Verification items for the finished model (mm, model axes). Face numbers are marked on the shaded views. A direction names the side the tool comes from. Give positions to 0.01 mm unless a question says otherwise; leave off trailing zeros. Loops run counter-clockwise (first coordinate to the right, second up) from the corner with the lowest first, then second, coordinate; pieces in that order, holes last. Notation, with made-up numbers: M 33,-6.75 L 72,-6.75 A15 ccw 72,10.25 Z; hole C 29.25,25.25 d1. An arc over 180 degrees is marked long. Answer in a Markdown table with one row per item.
```python
from build123d import *

# Parameters (mm, degrees)
SKETCH_1_W          = 30
SKETCH_1_H          = 25
SKETCH_1_W_2        = 28
SKETCH_1_H_2        = 23
EXTRUDE_1_DEPTH     = 27.5
SKETCH_2_R          = 1.5
CUT_EXTRUDE_1_DEPTH = 70
SKETCH_3_R          = 1.5
CUT_EXTRUDE_2_DEPTH = 20
SKETCH_4_R          = 1.5
CUT_EXTRUDE_3_DEPTH = 20


with BuildPart() as part:
    # 草图1 → 凸台-拉伸1 (new, symmetric)
    with BuildSketch(Plane.XY):
        Rectangle(SKETCH_1_W, SKETCH_1_H)
        Rectangle(SKETCH_1_W_2, SKETCH_1_H_2, mode=Mode.SUBTRACT)
    extrude(amount=EXTRUDE_1_DEPTH, both=True)

    # 草图2 → 切除-拉伸1 (cut)
    with BuildSketch(Plane(origin=(0, 12.5, 0), x_dir=(1, 0, 0), z_dir=(0, 1, 0))):
        with Locations(Location((0, 20, 0), (0, 0, 270))):
            Circle(SKETCH_2_R)
        with Locations(Location((0, -20, 0), (0, 0, 270))):
            Circle(SKETCH_2_R)
    extrude(amount=-CUT_EXTRUDE_1_DEPTH, mode=Mode.SUBTRACT)

    # 草图3 → 切除-拉伸2 (cut)
    with BuildSketch(Plane(origin=(-14, 0, 0), x_dir=(0, 0, -1), z_dir=(1, 0, 0))):
        Circle(SKETCH_3_R)
        with Locations((-23.5, 0)):
            Circle(SKETCH_3_R)
        with Locations((23.5, 0)):
            Circle(SKETCH_3_R)
    extrude(amount=-CUT_EXTRUDE_2_DEPTH, mode=Mode.SUBTRACT)

    # 草图4 → 切除-拉伸3 (cut)
    with BuildSketch(Plane(origin=(15, 0, 0), x_dir=(0, 0, -1), z_dir=(1, 0, 0))):
        with Locations((15, 0)):
            Circle(SKETCH_4_R)
        with Locations((-15, 0)):
            Circle(SKETCH_4_R)
    extrude(amount=-CUT_EXTRUDE_3_DEPTH, mode=Mode.SUBTRACT)


solid = part.part
```
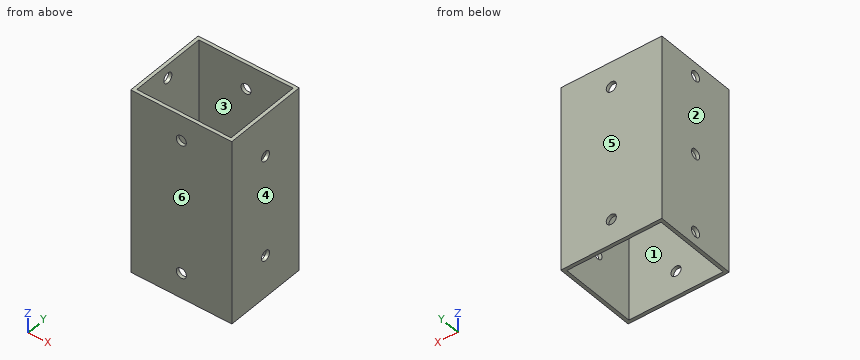
Item 1: Sectioned sample at B-B (z = -10). Record the cut outline in (x, y), and give its area (3 significant figures).
Reported:
| item | result |
|---|---|
| outline | M -15,-12.5 L 15,-12.5 L 15,12.5 L -15,12.5 Z; hole M -14,-11.5 L 14,-11.5 L 14,11.5 L -14,11.5 Z |
| area | 106 mm^2 |
Item 2: Sectioned sample at C-C (x = 5.5). Record the cut outline in (y, z), and give its area (3 significant figures).
Reported:
| item | result |
|---|---|
| outline | M -12.5,-27.5 L -11.5,-27.5 L -11.5,27.5 L -12.5,27.5 Z; M 11.5,-27.5 L 12.5,-27.5 L 12.5,27.5 L 11.5,27.5 Z |
| area | 110 mm^2 |
Item 3: Scan lines: L1, parallel to Y at x = -14.75, z = -23.5; L2, parallel to Y at x = 2, z = 12.5; L3, parallel to X at y = -8.25, z = -6. Record each from-to range of solid material in increasing order. Write a range as [from, to].
Reported:
| item | result |
|---|---|
| L1 | y = [-12.5, -1.5], [1.5, 12.5] |
| L2 | y = [-12.5, -11.5], [11.5, 12.5] |
| L3 | x = [-15, -14], [14, 15] |
Item 4: Go/stop test with a flat-tipped pin: pin 1 (1.8 mm diameter, centred on y = 0, z = 23.5, fed in from -X). Record where the tip stops, or that it passes through.
Reported:
| item | result |
|---|---|
| pin 1 | stops at x = 14 |
Item 5: Sectioned sample at A-A (y = 10). Record the cut outline in (x, z).
Reported:
| item | result |
|---|---|
| outline | M -15,-27.5 L -14,-27.5 L -14,27.5 L -15,27.5 Z; M 14,-27.5 L 15,-27.5 L 15,27.5 L 14,27.5 Z |
Item 6: Tool access check on the marked faces 1 and 2. Record the directions out of +Z, -Z, +X, -X, +Y, -Y that give a thin tool (end or side, any length) a straight path to the whole face; none if there is none.
Reported:
| item | result |
|---|---|
| face 1 | +Z, -Z |
| face 2 | +Z, -Z, -X, +Y, -Y |
Item 7: Sectioned sample at D-D (z = 20). Record the cut outline in (x, y).
Reported:
| item | result |
|---|---|
| outline | M -15,-12.5 L -1.5,-12.5 L -1.5,-11.5 L -14,-11.5 L -14,11.5 L -1.5,11.5 L -1.5,12.5 L -15,12.5 Z; M 1.5,-12.5 L 15,-12.5 L 15,12.5 L 1.5,12.5 L 1.5,11.5 L 14,11.5 L 14,-11.5 L 1.5,-11.5 Z |
Item 8: Release check for a two-part mould opening along Y. For the marked faces 3, 4, 5 and 6 record: released by +Y, released by -Y, zero draft, split by the parting line, or undercut.
Reported:
| item | result |
|---|---|
| face 3 | undercut |
| face 4 | zero draft |
| face 5 | released by +Y |
| face 6 | released by -Y |
